Design review of the part built by this model. Coordinates are the model's own, in mm. A direction names the side the tool comes from. Coordinates: 2 decimals unless noted, no trailing zeros. Write each loop counter-clockwise with the first axis right and the second up, starting at its lowest first coordinate (ties: lowest second). Pieces come first, ordered by that corner, then holes. Notation, with made-up numbers: (-19.75, 60.5) - (11.25, 60.5) arc R21 cw to (11.25, 80.5) - close; hole circle Ø8 at (31, 67). An arc over 180 degrees is marked (long way). Answer as CSV lines item,"result". Start each with the question number.
Q1. We need section A-A (x = 19.5). Write out the cut boundary in (y, z) (3 decimals), plus the area to 3 significant figures.
Q2. Mouldability with a two-part tool opening along X and no side actions: class faces 3 (the face through (129.54, -2, 9)), 4 (the face through (-2, 139.065, 9)), 5 (the face through (139.065, -2, 9)), 6 (the face through (-139.065, -2, 9)) as pulls with the +X half, pulls with the -X half, needs draft (parallel to the pull), parting line crosses it, or undercut.
Q3. For line 1 along X through (y, z) = (-4.5, 17.75) (3 decimals), list the stretches that pass through material, from the lowest coordinate up. Write a range as [from, to].
Q4. Machinability: for faces 1 (the face through (-2, -129.54, 9)), 2 (the face through (-11, -133, 0)), which of the approach directions +Z, -Z, +X, -X, +Y, -Y give a long, thin tool a straight path to every point of the face, cutting with its end or side? Answer none if there is none.
Q5. We need section B-B (z = 10). Write out the cut boundary in (x, y) (3 decimals), plus the area to 3 significant figures.
from build123d import *

# Parameters (mm, degrees)
SKETCH1_W           = 278.13
SKETCH1_H           = 278.13
SKETCH1_W_2         = 259.08
SKETCH1_H_2         = 259.08
BOSS_EXTRUDE1_DEPTH = 19.05
FILLET1_R           = 2.54


with BuildPart() as part:
    # Sketch1 → Boss-Extrude1 (new body)
    with BuildSketch(Plane.XY):
        Rectangle(SKETCH1_W, SKETCH1_H)
        Rectangle(SKETCH1_W_2, SKETCH1_H_2, mode=Mode.SUBTRACT)
    extrude(amount=BOSS_EXTRUDE1_DEPTH)

    # Fillet1
    fillet1_edges = [part.edges().sort_by_distance(p)[0] for p in [
        (129.54, -129.54, 9.525),
        (129.54, 129.54, 9.525),
        (-129.54, 129.54, 9.525),
        (-129.54, -129.54, 9.525),
        (139.065, -139.065, 9.525),
        (-139.065, -139.065, 9.525),
        (-139.065, 139.065, 9.525),
        (139.065, 139.065, 9.525),
    ]]
    fillet(fillet1_edges, radius=FILLET1_R)


solid = part.part
Results list:
1,outline,"(-139.065, 0) - (-129.54, 0) - (-129.54, 19.05) - (-139.065, 19.05) - close; (129.54, 0) - (139.065, 0) - (139.065, 19.05) - (129.54, 19.05) - close"
1,area,"363 mm2"
2,face 3,"undercut"
2,face 4,"needs draft"
2,face 5,"pulls with the +X half"
2,face 6,"pulls with the -X half"
3,line 1,"x = [-139.065, -129.54], [129.54, 139.065]"
4,face 1,"+Z, -Z"
4,face 2,"-Z, +X, -X, +Y, -Y"
5,outline,"(-139.065, -136.525) arc R2.54 ccw to (-136.525, -139.065) - (136.525, -139.065) arc R2.54 ccw to (139.065, -136.525) - (139.065, 136.525) arc R2.54 ccw to (136.525, 139.065) - (-136.525, 139.065) arc R2.54 ccw to (-139.065, 136.525) - close; hole (-129.54, -127) arc R2.54 ccw to (-127, -129.54) - (127, -129.54) arc R2.54 ccw to (129.54, -127) - (129.54, 127) arc R2.54 ccw to (127, 129.54) - (-127, 129.54) arc R2.54 ccw to (-129.54, 127) - close"
5,area,"10,200 mm2"
